Part model, mm, in its own coordinate system. Face numbers are marked on the shaded views. Coordinates: 2 decimals unless noted, no trailing zeros. Order: outer loops, then holes, each group sorted by start corner. A loop starts at its lowest first (then second) coordinate and runs counter-clockwise, first axis right, second up.
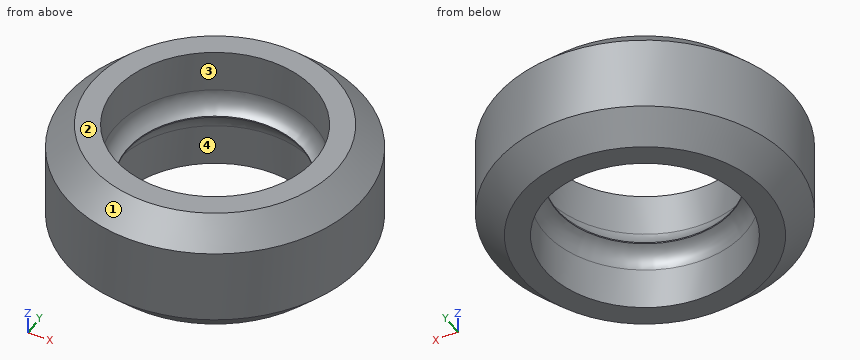
from build123d import *


# Not quite as in the source:
# - a fillet or chamfer that OpenCascade refuses, or shapes differently, is made with other operations: its cross-section is extruded or revolved along the edge and cut away or added


with BuildPart() as f1:
    # F0 (on Front) → F1 (revolve)
    with BuildSketch(Plane.XZ):
        Polygon((-7.1, 0.05), (-8.1, 0.05), (-8.1, 5.05), (-9.95, 5.05), (-12, 3), (-12, -3), (-9.95, -5.05), (-8.1, -5.05), (-8.1, -0.05), (-7.1, -0.05), align=None)
    revolve(axis=Axis((0, 0, 10.9107699245), (0, 0, -1)))

    # F2: fillet of radius 1.75 on 2 edges, made by hand

    # F2_s1 → F2_t2 (revolve)
    with BuildSketch(Plane.XZ):
        with BuildLine():
            ThreePointArc((-8.1, -1.6311388301), (-7.8290199458, -0.6957244834), (-7.1, -0.05))
            Line((-7.1, -0.05), (-7.115, -0.0183772234))
            ThreePointArc((-7.115, -0.0183772234), (-7.6, -0.015), (-8.1, -0.015))
            Line((-8.1, -0.015), (-8.135, -0.05))
            Line((-8.135, -0.05), (-8.135, -1.6311388301))
            Line((-8.135, -1.6311388301), (-8.1, -1.6311388301))
        make_face()
    revolve(axis=Axis((0, 0, -0.05), (0, 0, -1)))

    # F2_s3 → F2_t4 (revolve)
    with BuildSketch(Plane.XZ):
        with BuildLine():
            ThreePointArc((-7.1, 0.05), (-7.8290199458, 0.6957244834), (-8.1, 1.6311388301))
            Line((-8.1, 1.6311388301), (-8.135, 1.6311388301))
            Line((-8.135, 1.6311388301), (-8.135, 0.05))
            Line((-8.135, 0.05), (-8.1, 0.015))
            ThreePointArc((-8.1, 0.015), (-7.6, 0.015), (-7.115, 0.0183772234))
            Line((-7.115, 0.0183772234), (-7.1, 0.05))
        make_face()
    revolve(axis=Axis((0, 0, 0.05), (0, 0, -1)))


solid = f1.part
Q1. Cut at C-C on z = -2. Write the cut outline in (x, y).
Results list:
outline: circle Ø24 at (0, 0); hole circle Ø16.2 at (0, 0)
Q2. Mould opens along Y. For the marked faces 1, 2, 3 and 4 say: pulls with the +Y half, pulls with the -Y half, needs draft (parallel to the pull), parting line crosses it, or undercut.
Results list:
face 1: parting line crosses it
face 2: needs draft
face 3: undercut
face 4: undercut
Q3. Wall check: line 1 along Y through (x, z) = (0, 0); line 2 along Y through (x, z) = (0, 2.55); line 3 along X through (y, z) = (7, -3.75). Give the ranges that are in metal, low to high.
Results list:
line 1: y = -12 to -7.1, 7.1 to 12
line 2: y = -12 to -8.1, 8.1 to 12
line 3: x = -8.81 to -4.08, 4.08 to 8.81
Q4. Cut at A-A on y = 0. Write the cut outline in (x, z), and give its area (3 significant figures).
Results list:
outline: (-12, -3) - (-9.95, -5.05) - (-8.1, -5.05) - (-8.1, -1.63) arc R1.75 cw to (-7.1, -0.05) - (-7.1, 0.05) arc R1.75 cw to (-8.1, 1.63) - (-8.1, 5.05) - (-9.95, 5.05) - (-12, 3) - close; (7.1, -0.05) arc R1.75 cw to (8.1, -1.63) - (8.1, -5.05) - (9.95, -5.05) - (12, -3) - (12, 3) - (9.95, 5.05) - (8.1, 5.05) - (8.1, 1.63) arc R1.75 cw to (7.1, 0.05) - close
area: 72.4 mm2
Q5. Pin check, flat tips, straight feed: pin 1 Ø4 at (x, z) = (4.5, 4) entering from -Y; pin 2 Ø1.5 at (x, z) = (7, 2) entering from +Y; pin 3 Ø6 at (y, z) = (6, -2.5) entering from +X; pin 4 Ø8.5 at (x, y) = (0, 0) entering from +Z. Stop position of each tip, or through.
Results list:
pin 1: stops at y = -11.68
pin 2: stops at y = 10.24
pin 3: stops at x = 11.62
pin 4: passes through
